from build123d import *

# Parameters (mm, degrees)
SKETCH019_W     = 94
SKETCH019_H     = 94
SKETCH019_R     = 2.35
SKETCH019_R_2   = 1.65
PAD008_DEPTH    = 5
FILLET003_R     = 2
CHAMFER005_SIZE = 0.5
CHAMFER006_SIZE = 0.5


with BuildPart() as part:
    # Sketch019 → Pad008 (new body)
    with BuildSketch(Plane.YZ.offset(-35)):
        with Locations((0, 30.3506240158)):
            Rectangle(SKETCH019_W, SKETCH019_H)
        with Locations((0, 30.3506240158)):
            Circle(SKETCH019_R, mode=Mode.SUBTRACT)
        with Locations((-37, 67.3506240158)):
            Circle(SKETCH019_R_2, mode=Mode.SUBTRACT)
        with Locations((37, 67.3506240158)):
            Circle(SKETCH019_R_2, mode=Mode.SUBTRACT)
        with Locations((-37, -6.6493759842)):
            Circle(SKETCH019_R_2, mode=Mode.SUBTRACT)
        with Locations((37, -6.6493759842)):
            Circle(SKETCH019_R_2, mode=Mode.SUBTRACT)
        with Locations((0, -9.6493759842)):
            Circle(SKETCH019_R, mode=Mode.SUBTRACT)
    extrude(amount=-PAD008_DEPTH)

    # Fillet003
    fillet003_edges = [part.edges().sort_by_distance(p)[0] for p in [
        (-37.5, -47, -16.649376),
        (-37.5, -47, 77.350624),
        (-37.5, 47, 77.350624),
        (-37.5, 47, -16.649376),
    ]]
    fillet(fillet003_edges, radius=FILLET003_R)

    # Chamfer005
    chamfer005_edges = [part.edges().sort_by_distance(p)[0] for p in [
        (-35, -47, 30.350624),
        (-35, -46.414214, 76.764838),
        (-35, -46.414214, -16.06359),
        (-35, 0, 77.350624),
        (-35, 0, -16.649376),
        (-35, 46.414214, 76.764838),
        (-35, 46.414214, -16.06359),
        (-35, 47, 30.350624),
        (-35, -2.35, -9.649376),
        (-35, -2.35, 30.350624),
        (-35, 35.35, 67.350624),
        (-35, -38.65, 67.350624),
        (-35, 35.35, -6.649376),
        (-35, -38.65, -6.649376),
    ]]
    chamfer(chamfer005_edges, length=CHAMFER005_SIZE)

    # Chamfer006
    chamfer006_edges = [part.edges().sort_by_distance(p)[0] for p in [
        (-40, -47, 30.350624),
        (-40, -46.414214, 76.764838),
        (-40, -46.414214, -16.06359),
        (-40, 0, 77.350624),
        (-40, 0, -16.649376),
        (-40, 46.414214, 76.764838),
        (-40, 46.414214, -16.06359),
        (-40, 47, 30.350624),
        (-40, -2.35, -9.649376),
        (-40, -2.35, 30.350624),
        (-40, 35.35, 67.350624),
        (-40, -38.65, 67.350624),
        (-40, 35.35, -6.649376),
        (-40, -38.65, -6.649376),
    ]]
    chamfer(chamfer006_edges, length=CHAMFER006_SIZE)


solid = part.part
Work out the finished part from the listing and answer in its coordinate system (mm). Coordinates: 2 decimals unless noted, no trailing zeros. Write each loop counter-clockwise with the first axis right and the second up, starting at its lowest first coordinate (ties: lowest second). Pieces come first, ordered by that corner, then holes. Notation, with made-up numbers: M 8.25,-26.5 L 36.25,-26.5 A3 ccw 36.25,-21.5 Z; hole C 39,18 d2. An arc over 180 degrees is marked long. Answer as CSV lines item,"result". Start each with the question number.
Item 1: Consider L1, parallel to Z at x = -37.25, y = -37; L2, parallel to Y at x = -36.75, z = -7.5; L3, parallel to Z at x = -38.4, y = 0. Determine where each line is inside the solid, lowest interval first.
Item 2: Section A-A on y = 0 is taken. Write down the section's boundary in (x, z), and give its area (4 significant figures).
Item 3: Section B-B on y = 37 is taken. Write down the section's boundary in (x, z), and give its area (4 significant figures).
Item 4: Determine the mould class of faces 1 (the face through (-35.135, 46.144, 76.52)), 2 (the face through (-37, -47, 30)), 3 (the face through (-37.472, 1.263, -7.668)) for opening direction Y: released by +Y, released by -Y, zero draft, split by the parting line, or undercut.
Checks:
1,L1,"z = -16.65 to -8.3, -5 to 65.7, 69 to 77.35"
1,L2,"y = -47 to -38.41, -35.59 to -0.95, 0.95 to 35.59, 38.41 to 47"
1,L3,"z = -16.65 to -12, -7.3 to 28, 32.7 to 77.35"
2,outline,"M -40,-16.15 L -39.5,-16.65 L -35.5,-16.65 L -35,-16.15 L -35,-12.5 L -35.5,-12 L -39.5,-12 L -40,-12.5 Z; M -40,-6.8 L -39.5,-7.3 L -35.5,-7.3 L -35,-6.8 L -35,27.5 L -35.5,28 L -39.5,28 L -40,27.5 Z; M -40,33.2 L -39.5,32.7 L -35.5,32.7 L -35,33.2 L -35,76.85 L -35.5,77.35 L -39.5,77.35 L -40,76.85 Z"
2,area,"421.5 mm²"
3,outline,"M -40,-16.15 L -39.5,-16.65 L -35.5,-16.65 L -35,-16.15 L -35,-8.8 L -35.5,-8.3 L -39.5,-8.3 L -40,-8.8 Z; M -40,-4.5 L -39.5,-5 L -35.5,-5 L -35,-4.5 L -35,65.2 L -35.5,65.7 L -39.5,65.7 L -40,65.2 Z; M -40,69.5 L -39.5,69 L -35.5,69 L -35,69.5 L -35,76.85 L -35.5,77.35 L -39.5,77.35 L -40,76.85 Z"
3,area,"435.5 mm²"
4,face 1,"released by +Y"
4,face 2,"released by -Y"
4,face 3,"undercut"
